Source: three-view drawing plus pictorial views. Frame: mm from the lowest corner of the part. Give positions to 0.01 mm unless a question says otherwise; leave off trailing zeros. Order: outer loops, then holes, each group sorted by start corner. A loop starts at its lowest first (then second) coordinate and runs counter-clockwise, first axis right, second up. Notation, with made-up numbers: (73.5, 18.25) - (117.5, 18.25) arc R16 cw to (117.5, 39.25) - close; hole circle Ø2 at (46, 47). An arc over 180 degrees is marked (long way). Answer in a Markdown table with one row per item. Add a question column.
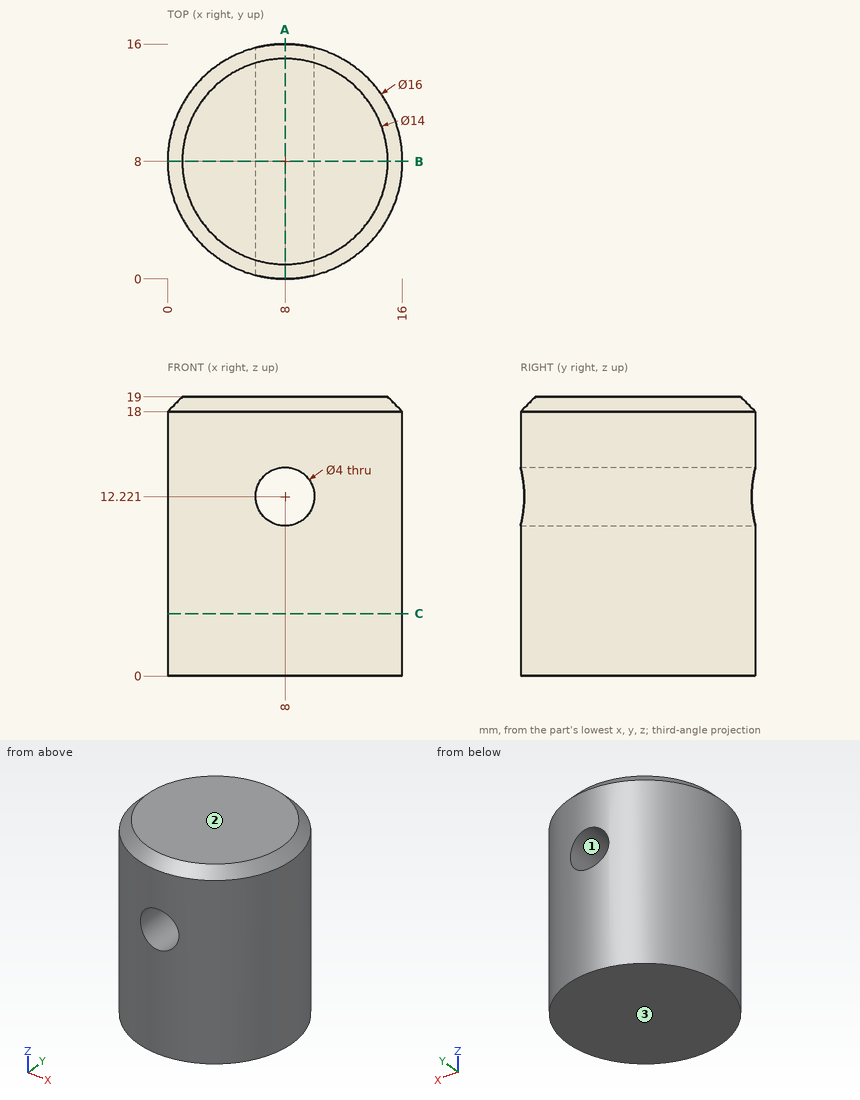
Q1. Section C-C, the plane z = 4.25. Return loops of the section in (x, y).
Q2. Section A-A, the plane x = 8. Return loops of the section in (y, z).
Q3. Line query: probe 1 along X at (y, z) = (6.5, 11.5) (1 decimal); probe 2 along X at (y, z) = (6.75, 12.5); probe 3 along Z at (x, y) = (9, 8.5). Output: solid intervals per line, ascending.
Q4. Pull-direction query (Z, two-part tool) for the marked faces 1, 2 and 3; classes: +Z half, -Z half, draft (parallel to the pull), parting line (faces both ways), or undercut.
Q5. Contact query for flat-ended pins moving along their axis: P1, Ø1, axis at y = 3.5, z = 5, coming from the -X side; P2, Ø8, axis at y = 10.5, z = 8.5, coming from the -X side; P3, Ø5, axis at x = 14, z = 7, coming from the +Y side; P4, Ø2.5, axis at x = 8, z = 12.22, coming from the -Y side. Output: stop coordinate, or through.
Q6. Section B-B, the plane y = 8. Return loops of the section in (x, z).
Computed:
| question | item | result |
|---|---|---|
| 1 | outline | circle Ø16 at (8, 8) |
| 2 | outline | (0, 0) - (16, 0) - (16, 10.22) - (0, 10.22) - close; (0, 14.22) - (16, 14.22) - (16, 18) - (15, 19) - (1, 19) - (0, 18) - close |
| 3 | probe 1 | x = 0.1 to 6.1, 9.9 to 15.9 |
| 3 | probe 2 | x = 0.1 to 6.02, 9.98 to 15.9 |
| 3 | probe 3 | z = 0 to 10.49, 13.95 to 19 |
| 4 | face 1 | undercut |
| 4 | face 2 | +Z half |
| 4 | face 3 | -Z half |
| 5 | P1 | stops at x = 1.07 |
| 5 | P2 | stops at x = 0 |
| 5 | P3 | stops at y = 15.19 |
| 5 | P4 | passes through |
| 6 | outline | (0, 0) - (16, 0) - (16, 18) - (15, 19) - (1, 19) - (0, 18) - close; hole circle Ø4 at (8, 12.22) |
